For this review, take the finished solid that the model builds, in its own axes (mm). A direction names the side the tool comes from. Coordinates: 2 decimals unless noted, no trailing zeros. Write each loop counter-clockwise with the first axis right and the second up, starting at its lowest first coordinate (ties: lowest second). Pieces come first, ordered by that corner, then holes.
1) We need section A-A on x = -28.5. Write out the cut boundary in (y, z), then the cut area to 3 significant figures.
2) For faces 4 (the face through (-26.7, -15.5, 29.6)), 5 (the face through (18.5, -9, 32)), 6 (the face through (-25, -18.5, 30)), list the 3-axis set-ups (+Z, -Z, +X, -X, +Y, -Y) from which the entire face can be reached by the end or side of a thin tool; tool diameter is ignored.
3) Insertion check: P1, Ø7.5, axis at x = 31, z = 16, coming from the +Y side; P2, Ø3, axis at x = 7.75, y = 13.42, coming from the -Z side; P3, Ø14, axis at x = 0, y = 7, coming from the +Z side; P4, Ø12, axis at y = 4.5, z = 36.5, coming from the +X side. Each pin has a flat end and moves straight along its axis. Give the tip position at first contact, or say it passes through.
4) We need section D-D on z = 33. Write out the cut boundary in (x, y).
5) To check wall thickness, follow line 1 along X through (y, z) = (-17, 54); line 2 along X through (y, z) = (0, 2.05); line 3 along X through (y, z) = (-13, 43). State the ranges of each line that lie inside material, in increasing order.
6) We need section C-C on y = 7. Write out the cut boundary in (x, z).
7) Mouldability with a two-part tool opening along Z and no side actions: class faces 1 (the face through (-27.235, -16.979, 54.806)), 2 (the face through (0, -4, 3)), 3 (the face through (21, -8, 30)) as pulls with the +Z half, pulls with the -Z half, needs draft (parallel to the pull), parting line crosses it, or undercut.
8) We need section B-B on z = 6. Write out the cut boundary in (x, y), then the cut area to 3 significant figures.
from build123d import *

# Parameters (mm, degrees)
SKETCH1_R           = 1.65
SKETCH1_R_2         = 6.15
BOSS_EXTRUDE1_DEPTH = 60
CUT_EXTRUDE1_DEPTH  = 57
SKETCH3_R           = 1.5
CUT_EXTRUDE2_DEPTH  = 79.919262541


with BuildPart() as part:
    # Sketch1 → Boss-Extrude1 (new body)
    with BuildSketch(Plane.XY):
        with BuildLine():
            Line((-21, 0), (-21, -15.5))
            Line((-21, -15.5), (-36, -15.5))
            Line((-36, -15.5), (-36, -18.5))
            Line((-36, -18.5), (36, -18.5))
            Line((36, -18.5), (36, -15.5))
            Line((36, -15.5), (21, -15.5))
            Line((21, -15.5), (21, 0))
            ThreePointArc((21, 0), (0, 21), (-21, 0))
        make_face()
        with Locations((-15.5, 0)):
            Circle(SKETCH1_R, mode=Mode.SUBTRACT)
        with Locations((-7.75, 13.423393759)):
            Circle(SKETCH1_R, mode=Mode.SUBTRACT)
        with Locations((7.75, 13.423393759)):
            Circle(SKETCH1_R, mode=Mode.SUBTRACT)
        with Locations((15.5, 0)):
            Circle(SKETCH1_R, mode=Mode.SUBTRACT)
        with Locations((7.75, -13.423393759)):
            Circle(SKETCH1_R, mode=Mode.SUBTRACT)
        with Locations((-7.75, -13.423393759)):
            Circle(SKETCH1_R, mode=Mode.SUBTRACT)
        with Locations((0, 7)):
            Circle(SKETCH1_R_2, mode=Mode.SUBTRACT)
    extrude(amount=BOSS_EXTRUDE1_DEPTH)

    # Sketch2 → Cut-Extrude1 (cut)
    with BuildSketch(Plane.XY.offset(60)):
        with BuildLine():
            Line((-18.5, 0), (-18.5, -18.5))
            Line((-18.5, -18.5), (18.5, -18.5))
            Line((18.5, -18.5), (18.5, 0))
            ThreePointArc((18.5, 0), (0, 18.5), (-18.5, 0))
        make_face()
    extrude(amount=-CUT_EXTRUDE1_DEPTH, mode=Mode.SUBTRACT)

    # Sketch3 → Cut-Extrude2 (cut, through all)
    with BuildSketch(Plane(origin=(0, -15.5, 0), x_dir=(1, 0, 0), z_dir=(0, 1, 0))):
        with Locations(Location((-28.5, -30, 0), (0, 0, 270))):
            Circle(SKETCH3_R)
        with Locations(Location((-28.5, -6, 0), (0, 0, 270))):
            Circle(SKETCH3_R)
        with Locations(Location((-28.5, -54, 0), (0, 0, 270))):
            Circle(SKETCH3_R)
        with Locations(Location((28.5, -54, 0), (0, 0, 90))):
            Circle(SKETCH3_R)
        with Locations(Location((28.5, -6, 0), (0, 0, 90))):
            Circle(SKETCH3_R)
        with Locations(Location((28.5, -30, 0), (0, 0, 90))):
            Circle(SKETCH3_R)
    extrude(amount=-CUT_EXTRUDE2_DEPTH, mode=Mode.SUBTRACT)


solid = part.part
Result:
1. outline: (-18.5, 0) - (-15.5, 0) - (-15.5, 4.5) - (-18.5, 4.5) - close; (-18.5, 7.5) - (-15.5, 7.5) - (-15.5, 28.5) - (-18.5, 28.5) - close; (-18.5, 31.5) - (-15.5, 31.5) - (-15.5, 52.5) - (-18.5, 52.5) - close; (-18.5, 55.5) - (-15.5, 55.5) - (-15.5, 60) - (-18.5, 60) - close
1. area: 153 mm2
2. face 4: +Z, -Z, -X, +Y
2. face 5: +Z, -Y
2. face 6: +Z, -Z, +X, -X, -Y
3. P1: stops at y = -15.5
3. P2: passes through
3. P3: stops at z = 3
3. P4: stops at x = 21
4. outline: (-36, -18.5) - (-18.5, -18.5) - (-18.5, 0) arc R18.5 cw to (18.5, 0) - (18.5, -18.5) - (36, -18.5) - (36, -15.5) - (21, -15.5) - (21, 0) arc R21 ccw to (-21, 0) - (-21, -15.5) - (-36, -15.5) - close
5. line 1: x = -36 to -30, -27 to -18.5, 18.5 to 27, 30 to 36
5. line 2: x = -21 to -17.15, -13.85 to 13.85, 17.15 to 21
5. line 3: x = -21 to -18.5, 18.5 to 21
6. outline: (-19.8, 0) - (-6.15, 0) - (-6.15, 3) - (-17.12, 3) - (-17.12, 60) - (-19.8, 60) - close; (6.15, 0) - (19.8, 0) - (19.8, 60) - (17.12, 60) - (17.12, 3) - (6.15, 3) - close
7. face 1: undercut
7. face 2: pulls with the +Z half
7. face 3: needs draft
8. outline: (-36, -18.5) - (-30, -18.5) - (-30, -15.5) - (-36, -15.5) - close; (-27, -18.5) - (-18.5, -18.5) - (-18.5, 0) arc R18.5 cw to (18.5, 0) - (18.5, -18.5) - (27, -18.5) - (27, -15.5) - (21, -15.5) - (21, 0) arc R21 ccw to (-21, 0) - (-21, -15.5) - (-27, -15.5) - close; (30, -18.5) - (36, -18.5) - (36, -15.5) - (30, -15.5) - close
8. area: 320 mm2
